Check sheet for the modelled part. Datum: model origin and axes. Units: mm. Give positions to 0.01 mm unless a question says otherwise; leave off trailing zeros. Write each loop counter-clockwise with the first axis right and the second up, starting at its lowest first coordinate (ties: lowest second). Pieces come first, ordered by that corner, then holes. Notation, with made-up numbers: M 37.5,9.25 L 90.5,9.25 A19 cw 90.5,15.25 Z; hole C 59.5,63 d7. An arc over 180 degrees is marked long. Write item = value, one per line. Start each with the question number.
1) Draft check along Z on faces 1 (the face through (-1, 1, 25)), 2 (the face through (20.765, -39.923, 8.662)), 3 (the face through (45.32, -14.27, 0.16)), 4 (the face through (-1, 1, 20)). Enter one of: pulls with the +Z half, pulls with the -Z half, needs draft (parallel to the pull), parting line crosses it, or undercut.
2) Sectioned sample at B-B, the plane z = 7. Record the cut outline in (x, y).
3) Scan lines: L1, parallel to Y at x = 0, z = 7.5; L2, parallel to Y at x = -5, z = 3.5; L3, parallel to Z at x = -24.5, y = 15. Record each from-to range of solid material in increasing order.
4) Sectioned sample at A-A, the plane x = 0. Record the cut outline in (y, z), then the cut area to 3 significant figures.
5) Gauge pin test, flat ends, axial feed: pin 1 (3 mm diameter, centred on x = 16.5, z = 20, fed in from -Y); pin 2 (1.5 mm diameter, centred on x = 19, y = -31, fed in from -Z); pin 3 (6 mm diameter, centred on y = 18, z = 6, fed in from -X). Record the tip position at first contact, or that the pin passes through.
from build123d import *

# Parameters (mm, degrees)
F0_R     = 50
F1_DEPTH = 25
F2_R     = 10
F3_T     = -5
F4_R     = 47.5
F4_R_2   = 45
F5_DEPTH = 2.5
F5_TAPER = -5


with BuildPart() as f1:
    # F0 (on Top) → F1 (new body)
    with BuildSketch(Plane.XY):
        Circle(F0_R)
    extrude(amount=F1_DEPTH)

    # F2
    f2_edges = [f1.edges().sort_by_distance(p)[0] for p in [
        (-50, 0, 25),
    ]]
    fillet(f2_edges, radius=F2_R)

    # F3
    f3_openings = [f1.faces().sort_by_distance(p)[0] for p in [
        (0, 0, 0),
    ]]
    offset(amount=F3_T, openings=f3_openings)

    # F4 (on face) → F5 (cut)
    with BuildSketch(Plane(origin=(0, 0, 0), x_dir=(1, 0, 0), z_dir=(0, 0, -1))):
        Circle(F4_R)
        Circle(F4_R_2, mode=Mode.SUBTRACT)
    extrude(amount=-F5_DEPTH, taper=F5_TAPER, mode=Mode.SUBTRACT)


solid = f1.part
Data:
q1.face_1 = pulls with the +Z half
q1.face_2 = needs draft
q1.face_3 = undercut
q1.face_4 = pulls with the -Z half
q2.outline = C 0,0 d100; hole C 0,0 d90
q3.L1 = -50 to -45, 45 to 50
q3.L2 = -49.75 to -44.72, 44.72 to 49.75
q3.L3 = 20 to 25
q4.outline = M -50,0 L -47.5,0 L -47.72,2.5 L -45,2.5 L -45,15 A5 cw -40,20 L 40,20 A5 cw 45,15 L 45,2.5 L 47.72,2.5 L 47.5,0 L 50,0 L 50,15 A10 ccw 40,25 L -40,25 A10 ccw -50,15 Z
q4.area = 655 mm2
q5.pin_1 = -46.71
q5.pin_2 = 20
q5.pin_3 = -47.7
